```python
from build123d import *

# Parameters (mm, degrees)
CYLINDER014_R          = 3
CYLINDER014_DEPTH      = 15
CYLINDER014_ROLL_ANGLE = 90
CYLINDER013_R          = 3
CYLINDER013_DEPTH      = 15
CYLINDER013_ROLL_ANGLE = 90
CYLINDER012_R          = 25
CYLINDER012_DEPTH      = 25
CYLINDER012_ROLL_ANGLE = 90


with BuildPart() as cylinder014:
    # Cylinder014 → Cylinder014 (new body)
    with BuildSketch(Plane.XY):
        Circle(CYLINDER014_R)
    extrude(amount=CYLINDER014_DEPTH)


with BuildPart() as cylinder014_1:
    # Cylinder014 roll: moved
    add(cylinder014.part.rotate(Axis((0, 0, 0), (1, 0, 0)), CYLINDER014_ROLL_ANGLE))


with BuildPart() as cylinder014_2:
    # Cylinder014 placement: moved
    add(cylinder014_1.part.moved(Location((258, 9, 130))))


with BuildPart() as cylinder013:
    # Cylinder013 → Cylinder013 (new body)
    with BuildSketch(Plane.XY):
        Circle(CYLINDER013_R)
    extrude(amount=CYLINDER013_DEPTH)


with BuildPart() as cylinder013_1:
    # Cylinder013 roll: moved
    add(cylinder013.part.rotate(Axis((0, 0, 0), (1, 0, 0)), CYLINDER013_ROLL_ANGLE))


with BuildPart() as cylinder013_2:
    # Cylinder013 placement: moved
    add(cylinder013_1.part.moved(Location((242, 9, 130))))


with BuildPart() as cut007:
    # Cylinder012 → Cylinder012 (new body)
    with BuildSketch(Plane.XY):
        Circle(CYLINDER012_R)
    extrude(amount=CYLINDER012_DEPTH)


with BuildPart() as cut007_1:
    # Cylinder012 roll: moved
    add(cut007.part.rotate(Axis((0, 0, 0), (1, 0, 0)), CYLINDER012_ROLL_ANGLE))


with BuildPart() as cut007_2:
    # Cylinder012 placement: moved
    add(cut007_1.part.moved(Location((250, 20, 130))))

    # Cut006: cut Cylinder013
    add(cylinder013_2.part, mode=Mode.SUBTRACT)

    # Cut007: cut Cylinder014
    add(cylinder014_2.part, mode=Mode.SUBTRACT)


with BuildPart() as cut007_3:
    # Cut007 placement: moved
    add(cut007_2.part.moved(Location((75, 0, -55))))


solid = cut007_3.part
```
Build history of the part. All positions in model axes, mm. A direction names the side the tool comes from. Give positions to 0.01 mm unless a question says otherwise; leave off trailing zeros. Loops run counter-clockwise (first coordinate to the right, second up) from the corner with the lowest first, then second, coordinate; pieces in that order, holes last.
Item 1: Which spindle directions (+Z, -Z, +X, -X, +Y, -Y) get a long thin tool onto all of the face, cutting with end or side? Do faces 1 (the face through (325, -5, 75)), 2 (the face through (335.77, 2.1, 73.85)). Say none if no direction does.
Answers follow:
face 1: +Z, -Z, +X, -X, -Y
face 2: -Y
Item 2: Slice it at C-C, the plane x = 332.5. List the corners of the cut face in (y, z).
Answers follow:
outline: (-5, 51.15) - (20, 51.15) - (20, 98.85) - (-5, 98.85) - (-5, 77.96) - (9, 77.96) - (9, 72.04) - (-5, 72.04) - close
Item 3: Pull direction Z, two halves, no side cores. Call faces 3 (the face through (333, 9, 75)), 4 (the face through (325, 20, 75)), 5 (the face through (348.846, 7.675, 82.509)): released by +Z, released by -Z, zero draft, split by the parting line, or undercut.
Answers follow:
face 3: undercut
face 4: zero draft
face 5: split by the parting line
Item 4: Flat gauge pins, fed straight in: pin 1 (5 mm diameter, centred on x = 333, z = 75, fed in from -Y); pin 2 (5 mm diameter, centred on y = 10.5, z = 90.5, fed in from -X); pin 3 (6 mm diameter, centred on x = 341, y = 4, fed in from -Z). Where does each tip first touch, or does it go through?
Answers follow:
pin 1: stops at y = 9
pin 2: stops at x = 303.65
pin 3: stops at z = 53.65
Item 5: Slice it at A-A, the plane z = 75. List the corners of the cut face in (x, y).
Answers follow:
outline: (300, -5) - (314, -5) - (314, 9) - (320, 9) - (320, -5) - (330, -5) - (330, 9) - (336, 9) - (336, -5) - (350, -5) - (350, 20) - (300, 20) - close
Item 6: Drill centre lines: line 1 (X direction, y = 4.25, z = 73.5); line 2 (Z direction, x = 317, y = 2); line 3 (Y direction, x = 332, z = 74). Where is each one in solid material? Low to high.
Answers follow:
line 1: x = 300.05 to 314.4, 319.6 to 330.4, 335.6 to 349.95
line 2: z = 51.31 to 72, 78 to 98.69
line 3: y = 9 to 20
Item 7: Slice it at B-B, the plane y = 4.75. List the corners of the cut face in (x, z).
Answers follow:
outline: circle Ø50 at (325, 75); hole circle Ø6 at (317, 75); hole circle Ø6 at (333, 75)
Item 8: Slice it at D-D, the plane y = 13.5. List the corners of the cut face in (x, z), and give its area (3 significant figures).
Answers follow:
outline: circle Ø50 at (325, 75)
area: 1,960 mm2
